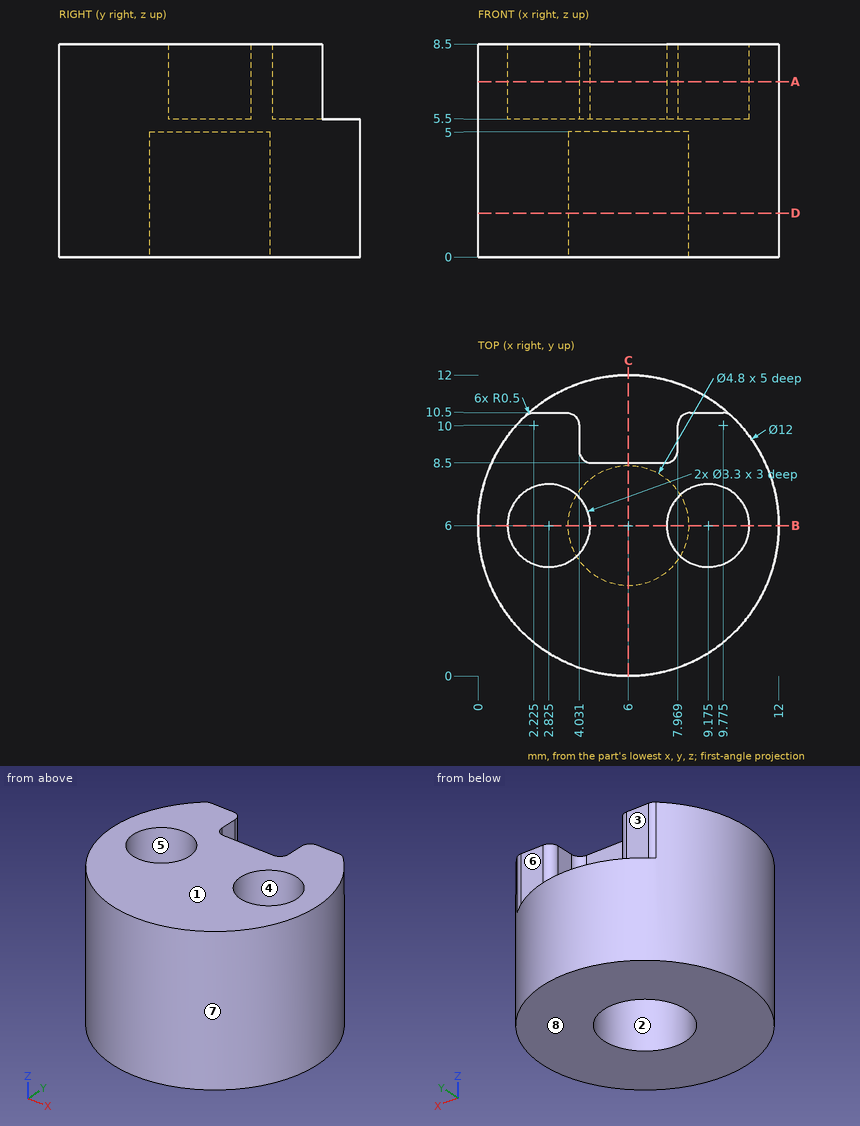
Can you work these out from the drawing? Everything is in mm from the part's minimum corner. A direction names the side the tool comes from. Round coordinates to 2 decimals unless told otherwise and drop trailing zeros. Loops run counter-clockwise (first coordinate to the right, second up) from the corner with the lowest first, then second, coordinate; pieces in that order, holes last. Notation, with made-up numbers: (24, 16.25) - (49, 16.25) arc R33 cw to (49, 46.25) - close; hole circle Ø2 at (29.25, 3.25). An arc over 180 degrees is marked (long way). Answer as CSV lines item,"result".
1. I want a section at B-B on y = 6. List the corners of the cut face in (x, z) for me (1 decimal), then the cut area to 3 significant figures.
Filled in:
outline,"(0, 0) - (3.6, 0) - (3.6, 5) - (8.4, 5) - (8.4, 0) - (12, 0) - (12, 8.5) - (10.8, 8.5) - (10.8, 5.5) - (7.5, 5.5) - (7.5, 8.5) - (4.5, 8.5) - (4.5, 5.5) - (1.2, 5.5) - (1.2, 8.5) - (0, 8.5) - close"
area,"58.2 mm^2"
2. I want a section at D-D on z = 1.75. List the corners of the cut face in (x, y) for me.
Filled in:
outline,"circle Ø12 at (6, 6); hole circle Ø4.8 at (6, 6)"
3. I want a section at C-C on x = 6. List the corners of the cut face in (y, z) for me.
Filled in:
outline,"(0, 0) - (3.6, 0) - (3.6, 5) - (8.4, 5) - (8.4, 0) - (12, 0) - (12, 5.5) - (8.5, 5.5) - (8.5, 8.5) - (0, 8.5) - close"
4. Please list where these lines run through material, in increasing order: line 1 along X through (y, z) = (6, 3.1); line 2 along Y through (x, z) = (11.5, 7) (1 decimal). Write a range as [from, to].
Filled in:
line 1,"x = [0, 3.6], [8.4, 12]"
line 2,"y = [3.6, 8.4]"
5. For pin 1 Ø1 at (x, y) = (10, 6.5) entering from +Z; pin 2 Ø2 at (y, z) = (9, 7) entering from +X; pin 3 Ø0.9 at (x, z) = (6, 6.5) entering from +Y, each with a flat end and sliding along its axis, tell me the tip position at first contact or that it passes through.
Filled in:
pin 1,"stops at z = 5.5"
pin 2,"stops at x = 11.66"
pin 3,"stops at y = 8.5"
6. I want a section at A-A on z = 7. Count the separate pieces of the cut face and the enclosed holes in it.
Filled in:
separate pieces,"1"
enclosed holes,"2"
7. We'd pull the mould along Y, two halves only. Please class the marked faces 5, 6, 7 and 8: +Y half, -Y half, draft (parallel to the pull), parting line (faces both ways), or undercut.
Filled in:
face 5,"undercut"
face 6,"+Y half"
face 7,"parting line"
face 8,"draft"
8. On a 3-axis mill with a long thin cutter (end or side, diameter ignored), from which of +Z, -Z, +X, -X, +Y, -Y can I reach the whole of each face in a straight line? I mean the marked faces 1, 2, 3 and 4. Say none if no direction works.
Filled in:
face 1,"+Z, +X, -X, +Y, -Y"
face 2,"-Z"
face 3,"+Z, +X, -X, +Y"
face 4,"+Z"
